```python
from build123d import *

# Parameters (mm, degrees)
F0_W     = 100
F0_H     = 95.3330463706
F1_DEPTH = 100
F2_W     = 100
F2_H     = 75.2818412601
F3_DEPTH = 40
F4_W     = 60
F4_H     = 15.817919746
F4_H_2   = 24.182080254
F5_DEPTH = 95.3340463706


with BuildPart() as f1:
    # F0 (on Top) → F1 (new body)
    with BuildSketch(Plane.XY):
        Rectangle(F0_W, F0_H)
    extrude(amount=F1_DEPTH)

    # F2 (on face) → F3 (cut)
    with BuildSketch(Plane.XY.offset(100)):
        with Locations((0, -10.0256025552)):
            Rectangle(F2_W, F2_H)
    extrude(amount=-F3_DEPTH, mode=Mode.SUBTRACT)

    # F4 (on face) → F5 (cut, through all)
    with BuildSketch(Plane.XZ.offset(47.6665231853)):
        with Locations((-5.323157385, -7.908959873)):
            Rectangle(F4_W, F4_H)
        with Locations((-5.323157385, 12.091040127)):
            Rectangle(F4_W, F4_H_2)
    extrude(amount=-F5_DEPTH, mode=Mode.SUBTRACT)


solid = f1.part
```
The listing builds one solid part. Answer for the finished solid, in the listing's coordinates (mm). A direction names the side the tool comes from. Give positions to 0.01 mm unless a question says otherwise; leave off trailing zeros. Write each loop counter-clockwise with the first axis right and the second up, starting at its lowest first coordinate (ties: lowest second). Pieces come first, ordered by that corner, then holes. Notation, with made-up numbers: M 19,58 L 60,58 A22 cw 60,97 Z; hole C -15.75,28 d11. An arc over 180 degrees is marked long. Write each question's results on one line, items separated by ' | '.
Q1. Section C-C, the plane x = 33 is taken. Write down the section's boundary in (y, z), then the cut area to 3 significant figures.
Output values:
outline: M -47.67,0 L 47.67,0 L 47.67,100 L 27.62,100 L 27.62,60 L -47.67,60 Z | area: 6,520 mm2
Q2. A tool of negligible diameter and unlimited length cuts with its end or side. For faces 1 (the flat face through (37, 1, 0)), 2 (the flat face through (-1, -9, 60)), 3 (the flat face through (-35.323, -1, 12)), from which of +Z, -Z, +X, -X, +Y, -Y can it reach the whole face along a straight path? Write none if from no direction.
Output values:
face 1: -Z, +X, -X, +Y, -Y | face 2: +Z, +X, -X, -Y | face 3: -Z, +Y, -Y
Q3. Section B-B, the plane y = 37 is taken. Write down the section's boundary in (x, z).
Output values:
outline: M -50,0 L -35.32,0 L -35.32,24.18 L 24.68,24.18 L 24.68,0 L 50,0 L 50,100 L -50,100 Z
Q4. Section D-D, the plane z = 70 is taken. Write down the section's boundary in (x, y), then the cut area to 3 significant figures.
Output values:
outline: M -50,27.62 L 50,27.62 L 50,47.67 L -50,47.67 Z | area: 2,010 mm2
Q5. Flat-ended cylindrical pins translate along their axes: P1, Ø3, axis at x = -12.5, y = 2, coming from the -Z side; P2, Ø20, axis at x = 5, z = 72.5, coming from the -Y side; P3, Ø2, axis at x = 16, y = 24, coming from the +Z side. Find the tip coordinate at first contact, or state that the pin passes through.
Output values:
P1: z = 24.18 | P2: y = 27.62 | P3: z = 60
Q6. For a pull along X with two mould halves and no side action, classify faces 4 (the flat face through (-1, -47.667, 36)), 5 (the flat face through (-50, 10, 38)), 6 (the flat face through (-6, -1, 24.182)) as released by +X, released by -X, zero draft, split by the parting line, or undercut.
Output values:
face 4: zero draft | face 5: released by -X | face 6: undercut
Q7. Consider L1, parallel to X at y = 22, z = 10; L2, parallel to Y at x = 46.5, z = 90.5; L3, parallel to Z at x = 8, y = 15. Determine where each line is inside the solid, lowest interval first. Write a range as from..to.
Output values:
L1: -50..-35.32, 24.68..50 | L2: 27.62..47.67 | L3: 24.18..60
Q8. Section A-A, the plane z = 21 is taken. Write down the section's boundary in (x, y).
Output values:
outline: M -50,-47.67 L -35.32,-47.67 L -35.32,47.67 L -50,47.67 Z; M 24.68,-47.67 L 50,-47.67 L 50,47.67 L 24.68,47.67 Z
